Autodesk Inventor part; units mm, degrees
ref_plane "YZ Plane" through (0, 0, 0) normal (1, 0, 0) x (0, 1, 0)
ref_plane "XZ Plane" through (0, 0, 0) normal (0, 1, 0) x (-1, 0, 0)
ref_plane "XY Plane" through (0, 0, 0) normal (0, 0, 1) x (1, 0, 0)
sketch "Sketch1" plane through (0, 0, 0) normal (0, 0, 1) x (1, 0, 0)
  line L0 (-50.8, -8.89) -> (50.8, -8.89)
  line L1 (50.8, -8.89) -> (50.8, 8.89)
  line L2 (50.8, 8.89) -> (-50.8, 8.89)
  line L3 (-50.8, 8.89) -> (-50.8, -8.89)
  line L4 (-50.8, -8.89) -> (50.8, 8.89) construction
  line L5 (50.8, -8.89) -> (-50.8, 8.89) construction
  point P0 (0, 0)
  dimension "d18" = 17.78
  dimension "d19" = 101.6
extrude "Extrusion1" add sketch "Sketch1" along normal mid plane 5.08
sketch "Sketch4" plane through (0, 0, 0) normal (0, 0, 1) x (1, 0, 0)
  line L0 (-50.8, -8.89) -> (-50.8, 8.89) construction
  line L1 (-50.8, 8.89) -> (50.8, 8.89) construction
  line L2 (50.8, 8.89) -> (50.8, -8.89) construction
  line L3 (50.8, -8.89) -> (-50.8, -8.89) construction
  arc A0 (46.99, -6.35) -> (46.99, 6.35) centre (46.99, 0) ccw
  line L4 (46.99, 6.35) -> (46.99, -6.35)
  point P0 (0, 0)
  point P1 (50.8, 0)
  dimension "d20" = 6.35
  dimension "d21" = 3.81
revolve "Revolution2" cut sketch "Sketch4" angle 360 about axis through (46.99, 6.35, 0) along (0, -1, 0)
mirror "Mirror1" about plane through (0, 0, 0) normal (1, 0, 0) of "Revolution2"
properties part number "deltabot arm"
The model under review builds one solid part; all positions refer to its coordinate system, in mm. Give positions to 0.01 mm unless a question says otherwise; leave off trailing zeros. Order: outer loops, then holes, each group sorted by start corner. A loop starts at its lowest first (then second) coordinate and runs counter-clockwise, first axis right, second up. Notation, with made-up numbers: M 89,63 L 116,63 A8 ccw 116,70 Z; hole C 62,14.5 d6. An arc over 180 degrees is marked long. One line per question, with ' | ' between items. Start each with the question number.
1) Wall thickness on L1, parallel to Y at x = -44, z = 1.35; L2, parallel to X at y = 5.5, z = 0.25; L3, parallel to X at y = 2.25, z = 2.2: over which ranges is each line inside the solid? List them lowest first. Write a range as from..to.
2) Mouldability with a two-part tool opening along Y and no side actions: class faces 1 (the face through (1, 8.89, 0)), 2 (the face through (-1, -8.89, 0)), 3 (the face through (50.8, -7, 0)) as pulls with the +Y half, pulls with the -Y half, needs draft (parallel to the pull), parting line crosses it, or undercut.
3) Consider section B-B, the plane y = 1.25. Give the boundary of the cut face in (x, z).
4) Consider section A-A, the plane z = -1.4. Give the boundary of the cut face in (x, y).
Found:
1) L1: y = -8.89..-5.44, 5.44..8.89 | L2: x = -50.8..-50.15, -43.83..43.83, 50.15..50.8 | L3: x = -41.47..41.47
2) face 1: pulls with the +Y half | face 2: pulls with the -Y half | face 3: needs draft
3) outline: M -41.31,-2.54 L 41.31,-2.54 A6.23 cw 41.31,2.54 L -41.31,2.54 A6.23 cw Z
4) outline: M -50.8,-8.89 L 50.8,-8.89 L 50.8,-4.88 A6.19 cw long 50.8,4.88 L 50.8,8.89 L -50.8,8.89 L -50.8,4.88 A6.19 cw long -50.8,-4.88 Z
